Work out the finished part from the listing and answer in its coordinate system (mm). A direction names the side the tool comes from. Give positions to 0.01 mm unless a question says otherwise; leave off trailing zeros. Loops run counter-clockwise (first coordinate to the right, second up) from the corner with the lowest first, then second, coordinate; pieces in that order, holes last.
Autodesk Inventor part; units mm, degrees
ref_plane "YZ Plane" through (0, 0, 0) normal (1, 0, 0) x (0, 1, 0)
ref_plane "XZ Plane" through (0, 0, 0) normal (0, 1, 0) x (-1, 0, 0)
ref_plane "XY Plane" through (0, 0, 0) normal (0, 0, 1) x (1, 0, 0)
sketch "スケッチ1" plane through (0, 0, 0) normal (0, 0, 1) x (1, 0, 0)
  circle A0 centre (76.2014, 18) radius 1.25
  circle A1 centre (70, 2) radius 1.5
  circle A2 centre (71.5626, -13) radius 1.25
  circle A3 centre (71.5626, -13) radius 5
  arc A4 (72.7656, 23.9999) -> (68.1729, -16.6757) centre (85.3759, 1.979) ccw
  circle A5 centre (139.7986, 18) radius 1.25
  circle A6 centre (139.7986, 18) radius 6.914
  arc A7 (147.8271, -16.6757) -> (143.2344, 23.9999) centre (130.6241, 1.979) ccw
  circle A8 centre (146, 2) radius 1.5
  circle A9 centre (144.4374, -13) radius 5
  circle A10 centre (144.4374, -13) radius 1.25
  circle A11 centre (76.2014, 18) radius 6.914
  line L0 (82.9641, 16.5612) -> (76.4531, -14.0405)
  line L1 (133.0359, 16.5612) -> (139.5469, -14.0405)
  arc A12 (87.1691, 16.7068) -> (81.2992, 8.7363) centre (93.0365, 6.239) ccw
  arc A13 (87.1691, 16.7068) -> (87.5297, 19.9375) centre (86.1912, 18.4514) ccw
  arc A14 (87.5297, 19.9375) -> (77.288, 24.8281) centre (74.1449, 5.0766) ccw
  line L2 (108, 72.8318) -> (108, -27.6373) construction
  arc A15 (134.7008, 8.7363) -> (128.8309, 16.7068) centre (122.9635, 6.239) ccw
  arc A16 (138.712, 24.8281) -> (128.4703, 19.9375) centre (141.8551, 5.0766) ccw
  arc A17 (128.4703, 19.9375) -> (128.8309, 16.7068) centre (129.8088, 18.4514) ccw
  circle A18 centre (82.8568, 0.0761) radius 1.5
  circle A19 centre (133.1432, 0.0761) radius 1.75
  circle A20 centre (82.8568, 0.0761) radius 3
  arc A21 (81.3922, 9.1736) -> (84.3249, 2.6924) centre (87.2609, 7.9249) ccw
  arc A22 (83.1326, -2.9112) -> (77.8155, -7.6372) centre (83.6841, -8.8858) ccw
  arc A23 (131.6751, 2.6924) -> (134.6078, 9.1736) centre (128.7391, 7.9249) ccw
  circle A24 centre (133.1432, 0.0761) radius 3
  arc A25 (138.1845, -7.6372) -> (132.8674, -2.9112) centre (132.3159, -8.8858) ccw
  circle A26 centre (76.2014, 18) radius 1.5
  circle A27 centre (71.5626, -13) radius 1.5
  point P0 (0, 0)
  point P1 (0, 0)
  point P2 (81.3565, 8.9919)
  dimension "d0" = 8
  dimension "d1" = 2
  dimension "d2" = 12
  dimension "d3" = 20
  dimension "d4" = 10
  dimension "d5" = 6
  dimension "d6" = 6
  dimension "d7" = 6
  dimension "d10" = 2.5
  dimension "d11" = 3
  dimension "d12" = 3
  dimension "d13" = 3
  dimension "d14" = 3
extrude "押し出し1" add sketch "スケッチ1" along normal blind 3 contours A3 | A3 A4 A11 L0 | A11 | L0 A12 A21 A20 A22 | A14 A13 A12 A21 L0 A11 | A20
equation "\"d7\" = d6"
equation "\"d12\" = d11"
equation "\"d13\" = d11"
equation "\"d14\" = d11"
properties part number "アンノーン" material "アルミニウム 2014-T4"
Q1. Section D-D on y = -13 is taken. Give the vertices of the cut face in (x, z).
Q2. Given pin 1 (4 mm diameter, centred on x = 78.5, y = 13, fed in from -Z), flat-ended and moving along its own axis, determine where the tip first touches the part or whether it passes through.
Q3. Section C-C on y = 18 is taken. Give the vertices of the cut face in (x, z), plus the area to 3 significant figures.
Q4. Which of the six approach directions +Z, -Z, +X, -X, +Y, -Y give full straight-line access (tool end or side, diameter ignored) to faces 1 (the face through (83.467, 13.479, 1.479)), 2 (the face through (83.66, -1.19, 1.48))?
Q5. Determine the mould class of faces 3 (the face through (60.125, 4.495, 1.479)), 4 (the face through (74.924, 24.795, 1.479)), 5 (the face through (81.91, 5.21, 1.48)), 6 (the face through (74.703, 17.934, 1.479)) for opening direction X: +X half, -X half, draft (parallel to the pull), parting line (faces both ways), or undercut.
Q6. Section A-A on y = 1 is taken. Give the vertices of the cut face in (x, z), plus the area to 3 significant figures.
Q7. Section B-B on z = 1.25 is taken. Give the vertices of the cut face in (x, y), plus the area to 3 significant figures.
Q8. Consider line 1 along Y through (x, z) = (82.75, 0.45); line 2 along Y through (x, z) = (69.25, 2.5); line 3 along X through (y, z) = (3, 2.65). Determine where each line is inside the solid, lowest interval first.
Check result:
1. outline: (64.89, 0) - (70.06, 0) - (70.06, 3) - (64.89, 3) - close; (73.06, 0) - (76.67, 0) - (76.67, 3) - (73.06, 3) - close
2. pin 1: stops at z = 0
3. outline: (65.7, 0) - (74.7, 0) - (74.7, 3) - (65.7, 3) - close; (77.7, 0) - (88.14, 0) - (88.14, 3) - (77.7, 3) - close
3. area: 58.3 mm2
4. face 1: +Z, -Z, +X
4. face 2: +Z, -Z
5. face 3: -X half
5. face 4: parting line
5. face 5: +X half
5. face 6: undercut
6. outline: (60.02, 0) - (68.88, 0) - (68.88, 3) - (60.02, 3) - close; (71.12, 0) - (81.68, 0) - (81.68, 3) - (71.12, 3) - close; (84.04, 0) - (85.71, 0) - (85.71, 3) - (84.04, 3) - close
6. area: 63.3 mm2
7. outline: (68.17, -16.68) arc R5 ccw to (76.45, -14.04) - (77.82, -7.64) arc R6 cw to (83.13, -2.91) arc R3 ccw to (84.32, 2.69) arc R6 cw to (81.32, 8.73) - (81.39, 9.17) arc R12 cw to (87.17, 16.71) arc R2 ccw to (87.53, 19.94) arc R20 ccw to (77.29, 24.83) arc R6.91 ccw to (72.77, 24) arc R25.38 ccw to start; hole circle Ø3 at (70, 2); hole circle Ø3 at (71.56, -13); hole circle Ø3 at (76.2, 18); hole circle Ø3 at (82.86, 0.08)
7. area: 748 mm2
8. line 1: y = -2.96 to -1.42, 1.57 to 3.97, 12.42 to 23.13
8. line 2: y = -17.43 to 0.7, 3.3 to 21.57
8. line 3: x = 60.02 to 68.88, 71.12 to 83.83
